Work out the finished part from the listing and answer in its coordinate system (mm). Face numbers are marked on the shaded views. A direction names the side the tool comes from. Coordinates: 2 decimals unless noted, no trailing zeros. Loops run counter-clockwise (first coordinate to the right, second up) from the corner with the lowest first, then second, coordinate; pieces in that order, holes last. Notation, with made-up numbers: (17.25, 70.5) -> (41.25, 70.5) arc R9 ccw to (41.25, 86.5) -> close; hole circle Ø7 at (47, 45). An arc over 180 degrees is marked (long way). Use a Markdown table: item, result.
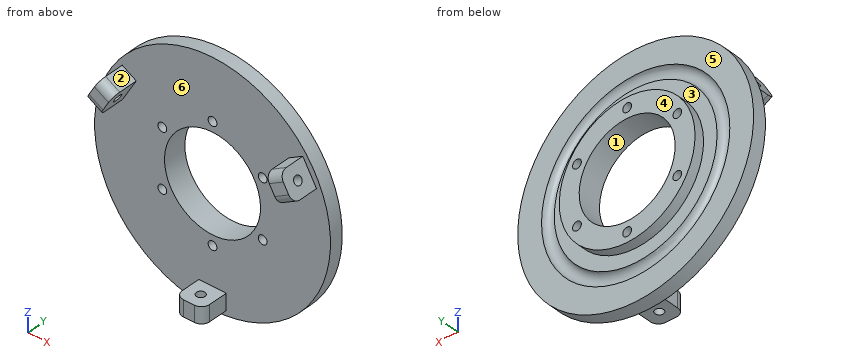
from build123d import *

# Parameters (mm, degrees)
SKETCH2_R                = 24.75
BOSS_EXTRUDE1_DEPTH      = 3.6
CUT_EXTRUDE1_DEPTH       = 62.416284485
CUT_EXTRUDE1_DEPTH_BACK  = 62.416284485
SKETCH3_R                = 17.5
CUT_EXTRUDE2_DEPTH       = 62.416284485
CUT_EXTRUDE2_DEPTH_BACK  = 62.416284485
SKETCH4_R                = 1.6
SKETCH5_W                = 10
SKETCH5_H                = 5.9
BOSS_EXTRUDE2_DEPTH      = 10
FILLET1_R                = 3
SKETCH6_R                = 1.55
CUT_EXTRUDE3_DEPTH       = 62.627915753
CIRPATTERN1_COUNT        = 3
FILLET1_OF_CIRPATTERN1_R = 3


with BuildPart() as part:
    # Sketch1 → Revolve1 (revolve)
    with BuildSketch(Plane.XY, mode=Mode.PRIVATE) as revolve1_sk:
        with BuildLine():
            Line((-34.322848467, 5), (-43, 5))
            Line((-43, 5), (-43, 0))
            Line((-43, 0), (0, 0))
            Line((0, 0), (0, 5))
            Line((0, 5), (-29.677151533, 5))
            ThreePointArc((-29.677151533, 5), (-32, 2.775), (-34.322848467, 5))
        make_face()
    revolve(revolve1_sk.sketch.rotate(Axis((0, 0, 0), (0, 1, 0)), 270), axis=Axis((0, 0, 0), (0, 1, 0)))

    # Sketch2 → Boss-Extrude1 (add)
    with BuildSketch(Plane(origin=(0, 5, 0), x_dir=(1, 0, 0), z_dir=(0, 1, 0))):
        with Locations(Location((0, 0, 0), (0, 0, 90))):
            Circle(SKETCH2_R)
    extrude(amount=BOSS_EXTRUDE1_DEPTH)

    # Sketch3 → Cut-Extrude1 (cut, two sides: drawn at the far end of the back side and taken through both)
    with BuildSketch(Plane(origin=(0, 8.6, 0), x_dir=(1, 0, 0), z_dir=(0, 1, 0)).offset(-CUT_EXTRUDE1_DEPTH_BACK)):
        with Locations(Location((0, 0, 0), (0, 0, 270))):
            Circle(SKETCH3_R)
    extrude(amount=CUT_EXTRUDE1_DEPTH + CUT_EXTRUDE1_DEPTH_BACK, mode=Mode.SUBTRACT)

    # Sketch4 → Cut-Extrude2 (cut, two sides: drawn at the far end of the back side and taken through both)
    with BuildSketch(Plane(origin=(0, 8.6, 0), x_dir=(1, 0, 0), z_dir=(0, 1, 0)).offset(-CUT_EXTRUDE2_DEPTH_BACK)):
        with Locations(Location((0, 21.125, 0), (0, 0, 270))):
            Circle(SKETCH4_R)
        with Locations(Location((18.294786655, 10.5625, 0), (0, 0, 270))):
            Circle(SKETCH4_R)
        with Locations(Location((18.294786655, -10.5625, 0), (0, 0, 270))):
            Circle(SKETCH4_R)
        with Locations(Location((0, -21.125, 0), (0, 0, 270))):
            Circle(SKETCH4_R)
        with Locations(Location((-18.294786655, -10.5625, 0), (0, 0, 270))):
            Circle(SKETCH4_R)
        with Locations(Location((-18.294786655, 10.5625, 0), (0, 0, 270))):
            Circle(SKETCH4_R)
    extrude(amount=CUT_EXTRUDE2_DEPTH + CUT_EXTRUDE2_DEPTH_BACK, mode=Mode.SUBTRACT)

    # Sketch5 → Boss-Extrude2 (add)
    with BuildSketch(Plane(origin=(0, 0, 0), x_dir=(1, 0, 0), z_dir=(0, 1, 0))):
        with Locations((0, 37.95)):
            Rectangle(SKETCH5_W, SKETCH5_H)
    boss_extrude2 = extrude(amount=-BOSS_EXTRUDE2_DEPTH)

    # Fillet1
    fillet1_edges = [part.edges().sort_by_distance(p)[0] for p in [
        (-5, -10, -37.95),
        (5, -10, -37.95),
    ]]
    fillet(fillet1_edges, radius=FILLET1_R)

    # Sketch6 → Cut-Extrude3 (cut, symmetric)
    with BuildSketch(Plane.XY):
        with Locations((0, -5)):
            Circle(SKETCH6_R)
    cut_extrude3 = extrude(amount=CUT_EXTRUDE3_DEPTH, both=True, mode=Mode.SUBTRACT)

    # CirPattern1: Boss-Extrude2, Cut-Extrude3 ×3 about axis
    cirpattern1_axis = Axis((0, 0, 0), (0, 1, 0))
    add([boss_extrude2.rotate(cirpattern1_axis, i * 360 / CIRPATTERN1_COUNT) for i in range(1, CIRPATTERN1_COUNT)])
    add([cut_extrude3.rotate(cirpattern1_axis, i * 360 / CIRPATTERN1_COUNT) for i in range(1, CIRPATTERN1_COUNT)], mode=Mode.SUBTRACT)

    # Fillet1 of CirPattern1
    fillet1_of_cirpattern1_edges = [part.edges().sort_by_distance(p)[0] for p in [
        (-30.365664074, -10, 23.305127019),
        (-35.365664074, -10, 14.644872981),
        (35.365664074, -10, 14.644872981),
        (30.365664074, -10, 23.305127019),
    ]]
    fillet(fillet1_of_cirpattern1_edges, radius=FILLET1_OF_CIRPATTERN1_R)


solid = part.part
Q1. Consider line 1 (X direction, y = 6.75, z = 0); line 2 (X direction, y = 1.5, z = 5.5); line 3 (Y direction, x = 21, z = 28). Determine where each line is inside the solid, lowest interval first. Write a range as [from, to].
Solved:
| item | result |
|---|---|
| line 1 | [-24.75, -17.5], [17.5, 24.75] |
| line 2 | [-42.65, -16.61], [16.61, 42.65] |
| line 3 | [0, 5] |
Q2. Section C-C on x = 0 is taken. State how many separate pieces and enclosed holes the cut face has, and give its area (3 significant figures).
Solved:
| item | result |
|---|---|
| separate pieces | 5 |
| enclosed holes | 0 |
| area | 277 mm² |
Q3. Section A-A on z = 0 is taken. Determine the outline of the cut face in (x, y) (3 decimals), and give its area (3 significant figures).
Solved:
| item | result |
|---|---|
| outline | (-43, 0) -> (-17.5, 0) -> (-17.5, 8.6) -> (-24.75, 8.6) -> (-24.75, 5) -> (-29.677, 5) arc R2.325 cw to (-34.323, 5) -> (-43, 5) -> close; (17.5, 0) -> (43, 0) -> (43, 5) -> (34.323, 5) arc R2.325 cw to (29.677, 5) -> (24.75, 5) -> (24.75, 8.6) -> (17.5, 8.6) -> close |
| area | 291 mm² |
Q4. Section B-B on y = -1.5 is taken. Determine the outline of the cut face in (x, z).
Solved:
| item | result |
|---|---|
| outline | (-37.92, 16.12) -> (-32.81, 13.17) -> (-27.81, 21.83) -> (-32.92, 24.78) -> close; (-5, -40.9) -> (5, -40.9) -> (5, -35) -> (-5, -35) -> close; (27.81, 21.83) -> (32.81, 13.17) -> (37.92, 16.12) -> (32.92, 24.78) -> close |
Q5. Determine the mould class of the marked faces 1, 2 and 3 for opening direction X: pulls with the +X half, pulls with the -X half, needs draft (parallel to the pull), parting line crosses it, or undercut.
Solved:
| item | result |
|---|---|
| face 1 | undercut |
| face 2 | undercut |
| face 3 | needs draft |
Q6. For the marked faces 4, 5 and 6, determine the directions among +Z, -Z, +X, -X, +Y, -Y from which every point of the face is accessible in a straight line to the end or side of a thin tool.
Solved:
| item | result |
|---|---|
| face 4 | +Z, -Z, +X, -X, +Y |
| face 5 | +Y |
| face 6 | -Y |
Q7. Given pin 1 Ø6 at (x, z) = (-22.5, 22) entering from -Y; pin 2 Ø4 at (x, y) = (28.5, 4) entering from +Z; pin 3 Ø3 at (x, y) = (-2, -2.5) entering from +Z, each flat-ended and moving along its own axis, determine where each tip first touches the part or whether it passes through.
Solved:
| item | result |
|---|---|
| pin 1 | y = 0 |
| pin 2 | z = 33.86 |
| pin 3 | z = -35 |
